Autodesk Inventor part; units mm, degrees
ref_plane "YZ Plane" through (0, 0, 0) normal (1, 0, 0) x (0, 1, 0)
ref_plane "XZ Plane" through (0, 0, 0) normal (0, 1, 0) x (-1, 0, 0)
ref_plane "XY Plane" through (0, 0, 0) normal (0, 0, 1) x (1, 0, 0)
sketch "Sketch1" plane through (0, 0, 0) normal (0, 1, 0) x (-1, 0, 0)
  line L0 (0, 0) -> (-6.35, 0)
  line L1 (-6.35, 0) -> (-6.35, -57.15)
  line L2 (0, -57.15) -> (0, 0)
  arc A0 (-1.5875, -57.15) -> (-4.7625, -57.15) centre (-3.175, -57.15) ccw
  line L3 (-6.35, -57.15) -> (-4.7625, -57.15)
  line L4 (-1.5875, -57.15) -> (0, -57.15)
  dimension "d0" = 6.35
  dimension "d1" = 57.15
  dimension "d2" = 3.175
revolve "Revolution1" add sketch "Sketch1" angle 360 about axis through (0, 0, 0) along (1, 0, 0)
sketch "Sketch2" plane through (6.35, 0, 0) normal (1, 0, 0) x (0, 0, -1)
  line L0 (-4.7625, 50.5763) -> (-4.7625, 4.7625)
  line L1 (-4.7625, -4.7625) -> (-4.7625, -50.5763)
  line L2 (4.7625, 50.5763) -> (4.7625, 4.7625)
  line L3 (4.7625, -4.7625) -> (4.7625, -50.5763)
  arc A0 (50.5763, 4.7625) -> (4.7625, 50.5763) centre (0, 0) ccw
  arc A1 (-4.7625, 50.5763) -> (-50.5763, 4.7625) centre (0, 0) ccw
  line L4 (-50.5763, 4.7625) -> (-4.7625, 4.7625)
  line L5 (4.7625, 4.7625) -> (50.5763, 4.7625)
  line L6 (-50.5763, -4.7625) -> (-4.7625, -4.7625)
  line L7 (4.7625, -4.7625) -> (50.5763, -4.7625)
  arc A2 (-50.5763, -4.7625) -> (-4.7625, -50.5763) centre (0, 0) ccw
  arc A3 (4.7625, -50.5763) -> (50.5763, -4.7625) centre (0, 0) ccw
extrude "Extrusion1" cut sketch "Sketch2" against normal blind 25.4
fillet "Fillet1" radius 3.175 12 edges at (3.175, 4.7625, 4.7625) (3.175, 4.7625, -4.7625) (3.175, -4.7625, -4.7625) (3.175, -4.7625, 4.7625) (3.175, -4.7625, -50.5763) (3.175, -50.5763, -4.7625) (3.175, -50.5763, 4.7625) (3.175, -4.7625, 50.5763) (3.175, 4.7625, 50.5763) (3.175, 50.5763, 4.7625) (3.175, 50.5763, -4.7625) (3.175, 4.7625, -50.5763)
sketch "Sketch3" plane through (6.35, 0, 0) normal (1, 0, 0) x (0, 0, -1)
  circle A0 centre (0, 0) radius 2.54
  dimension "d12" = 5.08
extrude "Extrusion2" cut sketch "Sketch3" against normal blind 25.4
chamfer "Chamfer1" distance 3.175 angle 45 48 edges at (6.35, -27.4482, -4.7625) (6.35, -5.6924, -5.6924) (6.35, -4.7625, -27.4482) (6.35, -5.888, -49.3838) (6.35, -35.921, -35.921) (6.35, -49.3838, -5.888) (6.35, -27.4482, 4.7625) (6.35, -49.3838, 5.888) (6.35, -35.921, 35.921) (6.35, -5.888, 49.3838) (6.35, -4.7625, 27.4482) (6.35, -5.6924, 5.6924) (6.35, 5.6924, 5.6924) (6.35, 27.4482, 4.7625) (6.35, 49.3838, 5.888) (6.35, 35.921, 35.921) (6.35, 5.888, 49.3838) (6.35, 4.7625, 27.4482) (6.35, 5.6924, -5.6924) (6.35, 4.7625, -27.4482) (6.35, 5.888, -49.3838) (6.35, 35.921, -35.921) (6.35, 49.3838, -5.888) (6.35, 27.4482, -4.7625) (0, 5.6924, 5.6924) (0, 4.7625, 27.4482) (0, 5.888, 49.3838) (0, 35.921, 35.921) (0, 49.3838, 5.888) (0, 27.4482, 4.7625) (0, -5.6924, 5.6924) (0, -27.4482, 4.7625) (0, -49.3838, 5.888) (0, -35.921, 35.921) (0, -5.888, 49.3838) (0, -4.7625, 27.4482) (0, -5.6924, -5.6924) (0, -4.7625, -27.4482) (0, -5.888, -49.3838) (0, -35.921, -35.921) (0, -49.3838, -5.888) (0, -27.4482, -4.7625) (0, 5.6924, -5.6924) (0, 27.4482, -4.7625) (0, 49.3838, -5.888) (0, 35.921, -35.921) (0, 5.888, -49.3838) (0, 4.7625, -27.4482)
properties part number "Wheel"
Could you check a few things on this model? Use its own coordinates, in mm. A direction names the side the tool comes from. Give positions to 0.01 mm unless a question says otherwise; leave off trailing zeros.
Item 1: For faces 3 (the face through (0.783, -2.513, 57.095)), 4 (the face through (4.43, 4.77, 4.84)), 5 (the face through (1.92, -4.84, -4.77)), which set-ups out of +Z, -Z, +X, -X, +Y, -Y let a thin tool reach every point of the face, with its end or its side?
Item 2: I need wall thicknesses on line 1 (Y direction, x = 5.25, z = 35.5); line 2 (Y direction, x = 2, z = -33.5); line 3 (Z direction, x = 1.5, y = 13.5). Which ranges of each line are inside material? Lowest first, please.
Item 3: I'm going to push flat-ended pins straight in: pin 1 (2 mm diameter, centred on x = 4.5, y = 32, fed in from +Z); pin 2 (1.5 mm diameter, centred on x = 3, z = 27, fed in from -Y); pin 3 (5 mm diameter, centred on y = -40, z = 35.5, fed in from +X); pin 4 (3 mm diameter, centred on x = 1.5, z = 41.5, fed in from +Y). Where does each tip first touch, or does it pass through?
Item 4: If we mould it in two halves opening along Y, with no side actions, what happens to faces 1 (the face through (4.785, -3.153, 27.175)), 2 (the face through (5.545, -2.513, 57.095))? For each: pulls with the +Y half, pulls with the -Y half, needs draft (parallel to the pull), parting line crosses it, or undercut.
Item 5: If we section it at C-C, the plane z = -48.5: Count the separate pieces of the cut face and the enclosed holes in it, plus the area to 3 significant figures.
Values:
1. face 3: +X, -X
1. face 4: +X
1. face 5: -X
2. line 1: y = -44.79 to -39.19, -2.69 to 2.69, 39.19 to 44.79
2. line 2: y = -44.98 to -39.74, -3.59 to 3.59, 39.74 to 44.98
2. line 3: z = -55.53 to -50.71, -3.09 to 3.09, 50.71 to 55.53
3. pin 1: stops at z = 47.99
3. pin 2: stops at y = -49.04
3. pin 3: stops at x = 6.35
3. pin 4: stops at y = 40.82
4. face 1: undercut
4. face 2: parting line crosses it
5. separate pieces: 3
5. enclosed holes: 0
5. area: 162 mm2
